Answer from the drawing. Dimensions are ordinates in mm from the lowest x, y and z of the part. A direction names the side the tool comes from. Give positions to 0.01 mm unless a question says otherwise; leave off trailing zeros. Write each loop counter-clockwise with the first axis right and the second up, starting at its lowest first coordinate (ties: lowest second). Pieces come first, ordered by that corner, then holes.
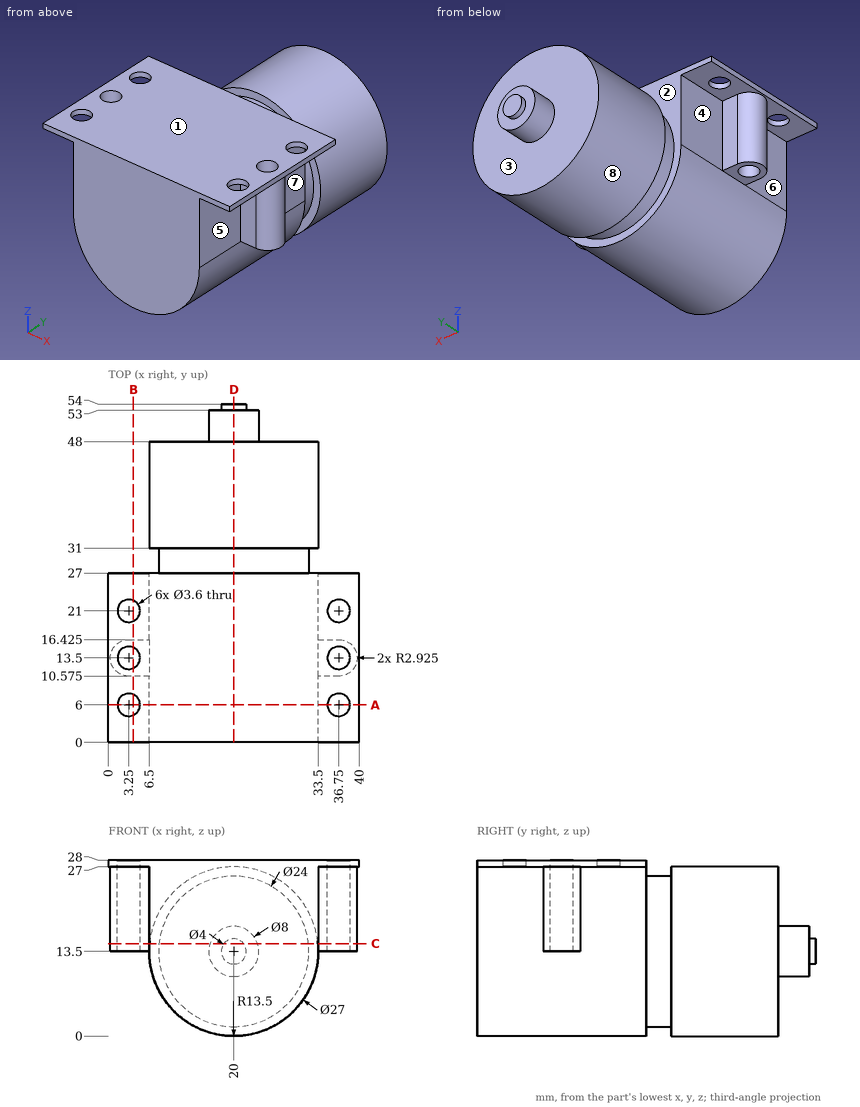
Item 1: Section C-C (z = 14.75) is taken. Give the number of separate pieces and of enclosed holes in the cut face, and give its area (3 significant figures).
Result set:
separate pieces: 1
enclosed holes: 2
area: 1,370 mm2
Item 2: Section B-B (x = 4) is taken. Write down the section's boundary in (y, z) (3 decimals).
Result set:
outline: (0, 27) - (4.364, 27) - (4.364, 28) - (0, 28) - close; (7.636, 27) - (10.575, 27) - (10.575, 13.5) - (11.864, 13.5) - (11.864, 28) - (7.636, 28) - close; (15.136, 13.5) - (16.425, 13.5) - (16.425, 27) - (19.364, 27) - (19.364, 28) - (15.136, 28) - close; (22.636, 27) - (27, 27) - (27, 28) - (22.636, 28) - close
Item 3: Each of these flat-tipped pins is pushed along its axis until it touches: pin 1 Ø3.5 at (x, z) = (4.5, 17) entering from -Y (3 decimals); pin 2 Ø2 at (x, y) = (24.5, 39.5) entering from -Z; pin 3 Ø8 at (x, y) = (22, 34) entering from +Z; pin 4 Ø3 at (x, y) = (36.75, 21) entering from +Z. Where does it stop, or does it pass through?
Result set:
pin 1: stops at y = 10.575
pin 2: stops at z = 0.46
pin 3: stops at z = 27
pin 4: passes through
Item 4: Find the intervals of material crossed by line 1 along Y through (x, z) = (3.25, 27.85); line 2 along Z through (x, y) = (19.5, 8); line 3 along Y through (x, z) = (29, 19.25), in increasing order.
Result set:
line 1: y = 0 to 4.2, 7.8 to 11.7, 15.3 to 19.2, 22.8 to 27
line 2: z = 0.01 to 28
line 3: y = 0 to 48
Item 5: Section A-A (y = 6) is taken. Write down the section's boundary in (x, z), and give its area (3 significant figures).
Result set:
outline: (0, 27) - (1.45, 27) - (1.45, 28) - (0, 28) - close; (5.05, 27) - (6.5, 27) - (6.5, 13.5) arc R13.5 ccw to (33.5, 13.5) - (33.5, 27) - (34.95, 27) - (34.95, 28) - (5.05, 28) - close; (38.55, 27) - (40, 27) - (40, 28) - (38.55, 28) - close
area: 684 mm2
Item 6: Which of the six approach directions +Z, -Z, +X, -X, +Y, -Y give full straight-line access (tool end or side, diameter ignored) to the marked faces 4, 5, 6, 7 and 8?
Result set:
face 4: -Z, -X, +Y
face 5: -Z, +X, -Y
face 6: -Z, -X, -Y
face 7: -Z, +X, +Y
face 8: +Y
Item 7: Determine the mould class of the marked faces 1, 2 and 3 for opening direction Y: pulls with the +Y half, pulls with the -Y half, needs draft (parallel to the pull), parting line crosses it, or undercut.
Result set:
face 1: needs draft
face 2: undercut
face 3: pulls with the +Y half
Item 8: Section D-D (x = 20) is taken. Write down the section's boundary in (y, z), and give its area (4 significant figures).
Result set:
outline: (0, 0) - (27, 0) - (27, 1.5) - (31, 1.5) - (31, 0) - (48, 0) - (48, 9.5) - (53, 9.5) - (53, 11.5) - (54, 11.5) - (54, 15.5) - (53, 15.5) - (53, 17.5) - (48, 17.5) - (48, 27) - (31, 27) - (31, 25.5) - (27, 25.5) - (27, 28) - (0, 28) - close
area: 1,355 mm2
